from build123d import *

# Parameters (mm, degrees)
CYLINDER067_R                        = 1.75
CYLINDER067_DEPTH                    = 22
CYLINDER067_PITCH_ANGLE              = 90
CYLINDER061_R                        = 1.25
CYLINDER061_DEPTH                    = 22
CYLINDER061_PITCH_ANGLE              = 90
CYLINDER062_R                        = 1.25
CYLINDER062_DEPTH                    = 22
CYLINDER062_PITCH_ANGLE              = 90
CYLINDER060_R                        = 1.25
CYLINDER060_DEPTH                    = 22
CYLINDER060_PITCH_ANGLE              = 90
CYLINDER059_R                        = 1.25
CYLINDER059_DEPTH                    = 22
CYLINDER059_PITCH_ANGLE              = 90
CYLINDER065_R                        = 1.25
CYLINDER065_DEPTH                    = 22
CYLINDER065_PITCH_ANGLE              = 90
CYLINDER066_R                        = 1.25
CYLINDER066_DEPTH                    = 22
CYLINDER066_PITCH_ANGLE              = 90
CYLINDER064_R                        = 1.25
CYLINDER064_DEPTH                    = 22
CYLINDER064_PITCH_ANGLE              = 90
CYLINDER063_R                        = 1.25
CYLINDER063_DEPTH                    = 22
CYLINDER063_PITCH_ANGLE              = 90
FUSION047_ROLL_ANGLE                 = 34
FUSION047_PLACEMENT_ANGLE            = -90
CYLINDER058_R                        = 3
CYLINDER058_DEPTH                    = 22
CYLINDER058_PITCH_ANGLE              = 90
CYLINDER057_R                        = 3
CYLINDER057_DEPTH                    = 13
CYLINDER057_ROLL_ANGLE               = 90
CYLINDER056_R                        = 10
CYLINDER056_DEPTH                    = 10
CYLINDER056_ROLL_ANGLE               = 90
PAD007_DEPTH                         = 34
PAD005_DEPTH                         = 42
CHAMFER104_SIZE                      = 1
CLONE020_PLACEMENT_ANGLE             = -90
PART_MIRRORING007012_PLACEMENT_ANGLE = 180


with BuildPart() as cilindro011:
    # Cylinder067 → Cylinder067 (new body)
    with BuildSketch(Plane.XY):
        Circle(CYLINDER067_R)
    extrude(amount=CYLINDER067_DEPTH)


with BuildPart() as cilindro011_1:
    # Cylinder067 pitch: moved
    add(cilindro011.part.rotate(Axis((0, 0, 0), (0, 1, 0)), CYLINDER067_PITCH_ANGLE))


with BuildPart() as cilindro011_2:
    # Cylinder067 placement: moved
    add(cilindro011_1.part.moved(Location((-4.75, -32, 125.75))))


with BuildPart() as cilindro005:
    # Cylinder061 → Cylinder061 (new body)
    with BuildSketch(Plane.XY):
        Circle(CYLINDER061_R)
    extrude(amount=CYLINDER061_DEPTH)


with BuildPart() as cilindro005_1:
    # Cylinder061 pitch: moved
    add(cilindro005.part.rotate(Axis((0, 0, 0), (0, 1, 0)), CYLINDER061_PITCH_ANGLE))


with BuildPart() as cilindro005_2:
    # Cylinder061 placement: moved
    add(cilindro005_1.part.moved(Location((20.25, -38, 124.25))))


with BuildPart() as cilindro006:
    # Cylinder062 → Cylinder062 (new body)
    with BuildSketch(Plane.XY):
        Circle(CYLINDER062_R)
    extrude(amount=CYLINDER062_DEPTH)


with BuildPart() as cilindro006_1:
    # Cylinder062 pitch: moved
    add(cilindro006.part.rotate(Axis((0, 0, 0), (0, 1, 0)), CYLINDER062_PITCH_ANGLE))


with BuildPart() as cilindro006_2:
    # Cylinder062 placement: moved
    add(cilindro006_1.part.moved(Location((20.25, -26, 127.25))))


with BuildPart() as cilindro004:
    # Cylinder060 → Cylinder060 (new body)
    with BuildSketch(Plane.XY):
        Circle(CYLINDER060_R)
    extrude(amount=CYLINDER060_DEPTH)


with BuildPart() as cilindro004_1:
    # Cylinder060 pitch: moved
    add(cilindro004.part.rotate(Axis((0, 0, 0), (0, 1, 0)), CYLINDER060_PITCH_ANGLE))


with BuildPart() as cilindro004_2:
    # Cylinder060 placement: moved
    add(cilindro004_1.part.moved(Location((20.25, -30, 118.75))))


with BuildPart() as fusion046:
    # Cylinder059 → Cylinder059 (new body)
    with BuildSketch(Plane.XY):
        Circle(CYLINDER059_R)
    extrude(amount=CYLINDER059_DEPTH)


with BuildPart() as fusion046_1:
    # Cylinder059 pitch: moved
    add(fusion046.part.rotate(Axis((0, 0, 0), (0, 1, 0)), CYLINDER059_PITCH_ANGLE))


with BuildPart() as fusion046_2:
    # Cylinder059 placement: moved
    add(fusion046_1.part.moved(Location((20.25, -34, 132.75))))

    # Fusion046: union Cilindro005, Cilindro006, Cilindro004
    add(cilindro005_2.part)
    add(cilindro006_2.part)
    add(cilindro004_2.part)


with BuildPart() as cilindro009:
    # Cylinder065 → Cylinder065 (new body)
    with BuildSketch(Plane.XY):
        Circle(CYLINDER065_R)
    extrude(amount=CYLINDER065_DEPTH)


with BuildPart() as cilindro009_1:
    # Cylinder065 pitch: moved
    add(cilindro009.part.rotate(Axis((0, 0, 0), (0, 1, 0)), CYLINDER065_PITCH_ANGLE))


with BuildPart() as cilindro009_2:
    # Cylinder065 placement: moved
    add(cilindro009_1.part.moved(Location((20.25, -38, 124.25))))


with BuildPart() as cilindro010:
    # Cylinder066 → Cylinder066 (new body)
    with BuildSketch(Plane.XY):
        Circle(CYLINDER066_R)
    extrude(amount=CYLINDER066_DEPTH)


with BuildPart() as cilindro010_1:
    # Cylinder066 pitch: moved
    add(cilindro010.part.rotate(Axis((0, 0, 0), (0, 1, 0)), CYLINDER066_PITCH_ANGLE))


with BuildPart() as cilindro010_2:
    # Cylinder066 placement: moved
    add(cilindro010_1.part.moved(Location((20.25, -26, 127.25))))


with BuildPart() as cilindro008:
    # Cylinder064 → Cylinder064 (new body)
    with BuildSketch(Plane.XY):
        Circle(CYLINDER064_R)
    extrude(amount=CYLINDER064_DEPTH)


with BuildPart() as cilindro008_1:
    # Cylinder064 pitch: moved
    add(cilindro008.part.rotate(Axis((0, 0, 0), (0, 1, 0)), CYLINDER064_PITCH_ANGLE))


with BuildPart() as cilindro008_2:
    # Cylinder064 placement: moved
    add(cilindro008_1.part.moved(Location((20.25, -30, 118.75))))


with BuildPart() as fusion047:
    # Cylinder063 → Cylinder063 (new body)
    with BuildSketch(Plane.XY):
        Circle(CYLINDER063_R)
    extrude(amount=CYLINDER063_DEPTH)


with BuildPart() as fusion047_1:
    # Cylinder063 pitch: moved
    add(fusion047.part.rotate(Axis((0, 0, 0), (0, 1, 0)), CYLINDER063_PITCH_ANGLE))


with BuildPart() as fusion047_2:
    # Cylinder063 placement: moved
    add(fusion047_1.part.moved(Location((20.25, -34, 132.75))))

    # Fusion047: union Cilindro009, Cilindro010, Cilindro008
    add(cilindro009_2.part)
    add(cilindro010_2.part)
    add(cilindro008_2.part)


with BuildPart() as fusion047_3:
    # Fusion047 roll: moved
    add(fusion047_2.part.rotate(Axis((0, 0, 0), (1, 0, 0)), FUSION047_ROLL_ANGLE))


with BuildPart() as fusion047_4:
    # Fusion047 placement: moved
    add(fusion047_3.part.moved(Location((114.107998, 21, 33.646227))).rotate(Axis((114.107998, 21, 33.646227), (0, 0, 1)), FUSION047_PLACEMENT_ANGLE))


with BuildPart() as cilindro002:
    # Cylinder058 → Cylinder058 (new body)
    with BuildSketch(Plane.XY):
        Circle(CYLINDER058_R)
    extrude(amount=CYLINDER058_DEPTH)


with BuildPart() as cilindro002_1:
    # Cylinder058 pitch: moved
    add(cilindro002.part.rotate(Axis((0, 0, 0), (0, 1, 0)), CYLINDER058_PITCH_ANGLE))


with BuildPart() as cilindro002_2:
    # Cylinder058 placement: moved
    add(cilindro002_1.part.moved(Location((20.25, -32, 125.75))))


with BuildPart() as cilindro001:
    # Cylinder057 → Cylinder057 (new body)
    with BuildSketch(Plane.XY):
        Circle(CYLINDER057_R)
    extrude(amount=CYLINDER057_DEPTH)


with BuildPart() as cilindro001_1:
    # Cylinder057 roll: moved
    add(cilindro001.part.rotate(Axis((0, 0, 0), (1, 0, 0)), CYLINDER057_ROLL_ANGLE))


with BuildPart() as cilindro001_2:
    # Cylinder057 placement: moved
    add(cilindro001_1.part.moved(Location((17.25, -6, 120))))


with BuildPart() as cilindro:
    # Cylinder056 → Cylinder056 (new body)
    with BuildSketch(Plane.XY):
        Circle(CYLINDER056_R)
    extrude(amount=CYLINDER056_DEPTH)


with BuildPart() as cilindro_1:
    # Cylinder056 roll: moved
    add(cilindro.part.rotate(Axis((0, 0, 0), (1, 0, 0)), CYLINDER056_ROLL_ANGLE))


with BuildPart() as cilindro_2:
    # Cylinder056 placement: moved
    add(cilindro_1.part.moved(Location((17.25, -4, 120))))


with BuildPart() as pad007:
    # Sketch012 → Pad007 (new body)
    with BuildSketch(Plane(origin=(3, -12, -1), x_dir=(0, 1, 0), z_dir=(1, 0, 0))):
        Polygon((-4.882067, 101.940956), (-4.882067, 138.559921), (-40.571098, 142.373672), (-40.571098, 120.688431), align=None)
    extrude(amount=PAD007_DEPTH)


with BuildPart() as right_shoulder:
    # Sketch010 → Pad005 (new body)
    with BuildSketch(Plane.YZ.offset(-1)):
        with BuildLine():
            Line((-35.729516, 116.76657), (-15.773906, 107.988197))
            Line((-15.773906, 107.988197), (-7.000344, 107.988197))
            Line((-7.000344, 107.988197), (-7.000344, 136.642965))
            Line((-7.000344, 136.642965), (-31.550963, 136.642965))
            ThreePointArc((-31.550963, 136.642965), (-41.706398, 128.400491), (-35.729516, 116.76657))
        make_face()
    extrude(amount=PAD005_DEPTH)

    # Cut085: cut Pad007
    add(pad007.part, mode=Mode.SUBTRACT)

    # Cut086: cut Cilindro
    add(cilindro_2.part, mode=Mode.SUBTRACT)

    # Cut087: cut Cilindro001
    add(cilindro001_2.part, mode=Mode.SUBTRACT)

    # Chamfer104
    chamfer104_edges = [right_shoulder.edges().sort_by_distance(p)[0] for p in [
        (-1, -7.000344, 122.315581),
    ]]
    chamfer(chamfer104_edges, length=CHAMFER104_SIZE)

    # Cut088: cut Cilindro002
    add(cilindro002_2.part, mode=Mode.SUBTRACT)

    # Cut089: cut Fusion047
    add(fusion047_4.part, mode=Mode.SUBTRACT)

    # Cut090: cut Fusion046
    add(fusion046_2.part, mode=Mode.SUBTRACT)

    # Cut091: cut Cilindro011
    add(cilindro011_2.part, mode=Mode.SUBTRACT)


with BuildPart() as right_shoulder_1:
    # Clone020 placement: moved
    add(right_shoulder.part.moved(Location((-275, 70, 2.5))).rotate(Axis((-275, 70, 2.5), (0, 0, 1)), CLONE020_PLACEMENT_ANGLE))


with BuildPart() as left_shoulder:
    # Part__Mirroring007012: instance of right-shoulder
    add(right_shoulder_1.part.mirror(Plane(origin=(0, 0, 0), x_dir=(1, 0, 0), z_dir=(0, 1, 0))))


with BuildPart() as left_shoulder_1:
    # Part__Mirroring007012 placement: moved
    add(left_shoulder.part.moved(Location((-478, 0, 0))).rotate(Axis((-478, 0, 0), (0, 0, 1)), PART_MIRRORING007012_PLACEMENT_ANGLE))


solid = left_shoulder_1.part
The model under review builds one solid part; all positions refer to its coordinate system, in mm. A direction names the side the tool comes from. Give positions to 0.01 mm unless a question says otherwise; leave off trailing zeros. Order: outer loops, then holes, each group sorted by start corner. A loop starts at its lowest first (then second) coordinate and runs counter-clockwise, first axis right, second up. Notation, with made-up numbers: (53.25, -2.5) -> (83.25, -2.5) arc R11 cw to (83.25, 17.5) -> close; hole circle Ø3 at (73.25, -37.75). An arc over 180 degrees is marked (long way). Write item = value, one per line. Start each with the question number.
(1) Take a section at A-A (z = 135.25). Write out the cut boundary in (x, y), plus the area to 3 significant figures.
(2) For pin 1 Ø2 at (x, z) = (-173, 121.25) entering from -Y; pin 2 Ø7 at (y, z) = (52.75, 122.5) entering from -X; pin 3 Ø5 at (y, z) = (40, 126) entering from +X; pin 4 Ø1.5 at (y, z) = (47.17, 117.82) entering from -X, all flat-tipped, find the tip position at first contact; note any pin that passes through.
(3) Tool access review of faces 1 (the cylindrical face through (-187.58, 54.96, 124.53)), 2 (the flat face through (-176, 33, 128)), 3 (the cylindrical face through (-171.891, 31.028, 120.673)): name each direction out of +Z, -Z, +X, -X, +Y, -Y from which nothing blocks a thin tool from reaching the whole face with its end or side.
(4) Take a section at C-C (y = 66.5). Write out the cut boundary in (x, z).
(5) For L1, parallel to Y at x = -179.5, z = 136.25; L2, parallel to Y at x = -186.95, z = 122.5; L3, parallel to X at y = 31.2, z = 128.25, list the stretches that pass through material, from the lowest coordinate up. Write a range as from..to.
(6) Take a section at B-B (x = -173.5). Write out the cut boundary in (y, z).
(7) Draft analysis for pull direction X (two halves, no side actions). For faces 4 (the flat face through (-186.81, 50.1, 110.67)), 5 (the flat face through (-176, 67, 128)), 6 (the cylindrical face through (-164, 31, 126)), state which applies: +X half, -X half, draft (parallel to the pull), parting line (faces both ways), or undercut.
Returned:
q1.outline = (-196, 29) -> (-170.25, 29) -> (-170.25, 33) -> (-186.12, 33) -> (-186.12, 67) -> (-163.35, 67) -> (-163.35, 71) -> (-195, 71) -> (-196, 70) -> close; (-167.75, 29) -> (-163.35, 29) -> (-163.35, 33) -> (-167.75, 33) -> close
q1.area = 587 mm²
q2.pin_1 = 67
q2.pin_2 = -189
q2.pin_3 = -186.12
q2.pin_4 = through
q3.face_1 = +X, -X
q3.face_2 = +Z, -Z, +X
q3.face_3 = -Y
q4.outline = (-196, 110.49) -> (-187.23, 110.49) -> (-186.12, 110.98) -> (-186.12, 139.14) -> (-196, 139.14) -> close
q5.L1 = 29..33, 67..71
q5.L2 = 29..49.75, 55.75..71
q5.L3 = -196..-174, -168..-161.08
q6.outline = (29, 116.53) -> (33, 116.53) -> (33, 120.1) -> (29, 120.1) -> close; (29, 122.4) -> (33, 122.4) -> (33, 126.59) -> (29, 126.59) -> close; (29, 129.91) -> (33, 129.91) -> (33, 139.14) -> (29, 139.14) -> close; (67, 116.53) -> (71, 116.53) -> (71, 139.14) -> (67, 139.14) -> close
q7.face_4 = +X half
q7.face_5 = draft
q7.face_6 = undercut
